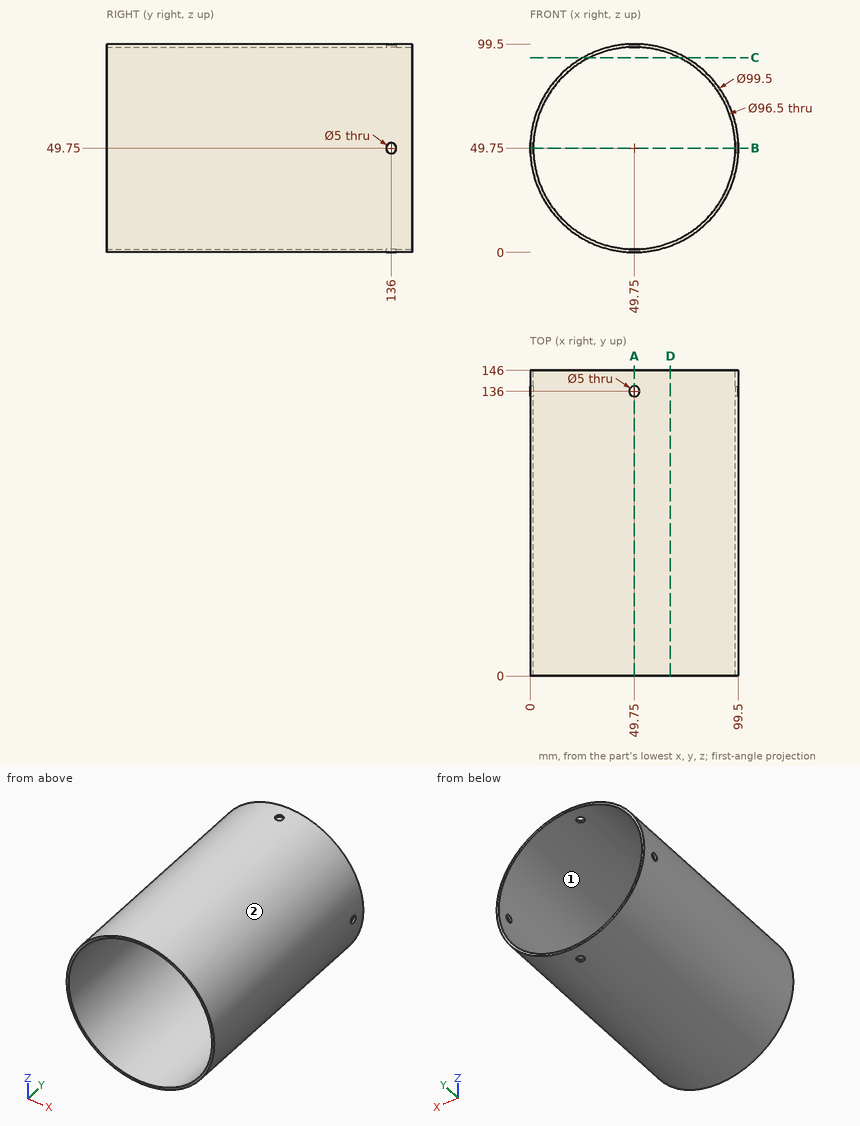
Geometry check sheet. Reference: drawing and pictorial views, mm from the part's lowest x, y, z. Round coordinates to 2 decimals unless told otherwise and drop trailing zeros. Order: outer loops, then holes, each group sorted by start corner. A loop starts at its lowest first (then second) coordinate and runs counter-clockwise, first axis right, second up. Notation, with made-up numbers: M -20,-11 L -13,-11 A15 ccw -13,7 Z; hole C 38.25,49.5 d8. An arc over 180 degrees is marked long. Write item = value, one per line.
Q1. Section check D-D (x = 67). Enter the section's corners in (y, z).
Answer block:
outline = M 0,3.09 L 146,3.09 L 146,4.69 L 0,4.69 Z; M 0,94.81 L 146,94.81 L 146,96.41 L 0,96.41 Z
Q2. Depth check by flat-ended pin: pin 1 Ø3 at (y, z) = (136, 49.75) entering from +X; pin 2 Ø1 at (y, z) = (131, 34.5) entering from -X; pin 3 Ø5 at (x, y) = (11.5, 78.5) entering from +Z; pin 4 Ø4 at (y, z) = (87, 35.5) entering from -X. Enter the tip coordinate at first touch or a pass-through.
Answer block:
pin_1 = through
pin_2 = 2.24
pin_3 = 84.35
pin_4 = 1.53
Q3. Section check C-C (z = 93). Enter the section's corners in (x, y), plus the area to 3 significant figures.
Answer block:
outline = M 25.16,0 L 28.36,0 L 28.36,146 L 25.16,146 Z; M 71.14,0 L 74.34,0 L 74.34,146 L 71.14,146 Z
area = 934 mm^2
Q4. Scan lines: line 1 (Z direction, x = 49, y = 92); line 2 (X direction, y = 67.5, z = 8.5); line 3 (Z direction, x = 75, y = 9.5). Record each from-to range of solid material in increasing order.
Answer block:
line_1 = 0.01 to 1.51, 97.99 to 99.49
line_2 = 21.94 to 24.72, 74.78 to 77.56
line_3 = 6.88 to 8.63, 90.87 to 92.62
Q5. Section check B-B (z = 49.75). Enter the section's corners in (x, y), plus the area to 3 significant figures.
Answer block:
outline = M 0,0 L 1.5,0 L 1.5,133.5 L 0,133.5 Z; M 0,138.5 L 1.5,138.5 L 1.5,146 L 0,146 Z; M 98,0 L 99.5,0 L 99.5,133.5 L 98,133.5 Z; M 98,138.5 L 99.5,138.5 L 99.5,146 L 98,146 Z
area = 423 mm^2
Q6. Release check for a two-part mould opening along X. For the marked faces 1 and 2 record: released by +X, released by -X, zero draft, split by the parting line, or undercut.
Answer block:
face_1 = undercut
face_2 = split by the parting line
Q7. Section check A-A (x = 49.75). Enter the section's corners in (y, z).
Answer block:
outline = M 0,0 L 133.5,0 L 133.5,1.5 L 0,1.5 Z; M 0,98 L 133.5,98 L 133.5,99.5 L 0,99.5 Z; M 138.5,0 L 146,0 L 146,1.5 L 138.5,1.5 Z; M 138.5,98 L 146,98 L 146,99.5 L 138.5,99.5 Z
